Verification items for this drawing (mm, ordinates from the low corner). Give positions to 0.01 mm unless a question says otherwise; leave off trailing zeros. Order: outer loops, then holes, each group sorted by start corner. A loop starts at its lowest first (then second) coordinate and runs counter-clockwise, first axis right, second up. Notation, with made-up numbers: M 74.5,-23 L 83.5,-23 A25 cw 83.5,9 Z; hole C -34.5,3.5 d5. An arc over 180 degrees is marked long. Answer as a JSON object with one key per item and string values.
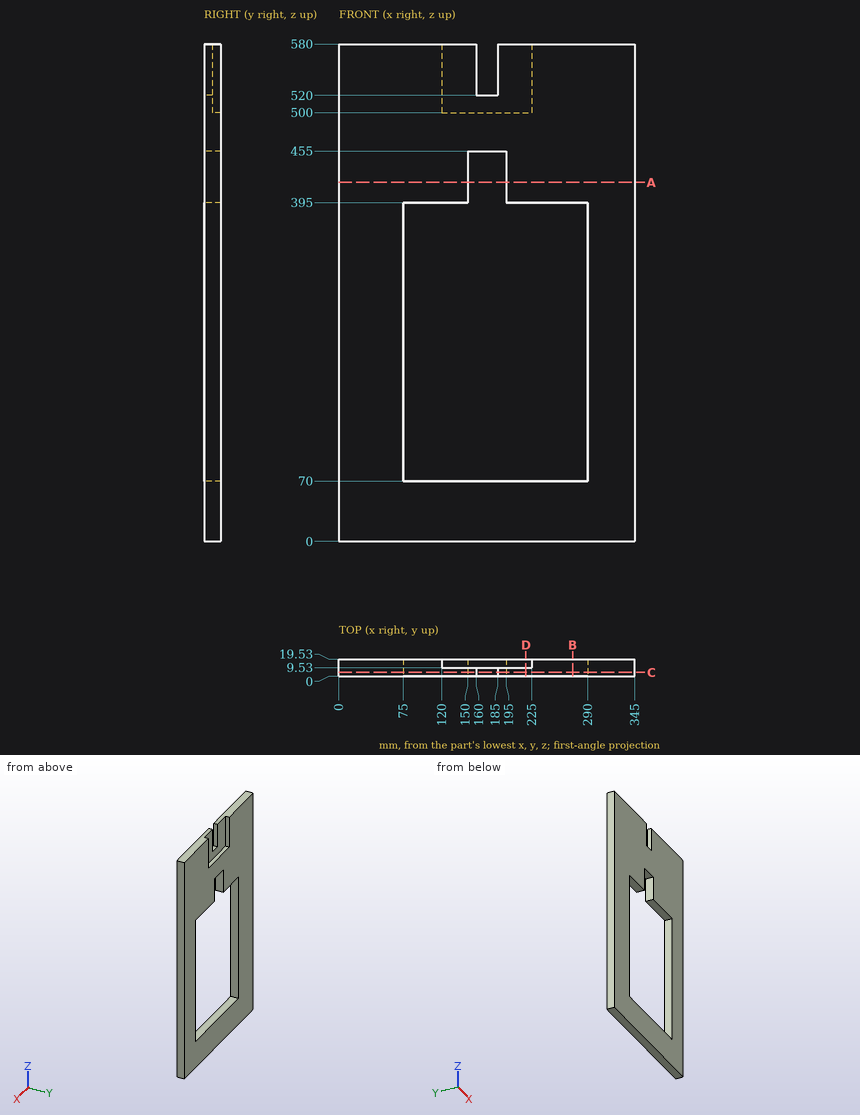
Q1. Material ranges on L1, parallel to Z at x = 204, y = 12.75; L2, parallel to Z at x = 90, y = 1; L3, parallel to X at y = 5, z = 333.5, recorded low to high.
Resolved:
{"L1": "z = 0 to 70, 395 to 500", "L2": "z = 0 to 70, 395 to 580", "L3": "x = 0 to 75, 290 to 345"}
Q2. Gauge pin test, flat ends, axial feed: pin 1 Ø5 at (x, y) = (169.5, 4) entering from +Z; pin 2 Ø6 at (x, y) = (224.5, 15.5) entering from +Z; pin 3 Ø24 at (x, z) = (162.5, 527.5) entering from +Y; pin 4 Ø3 at (x, y) = (163.5, 15) entering from +Z. Record the tip position at first contact, or that the pin passes through.
Resolved:
{"pin 1": "stops at z = 520", "pin 2": "stops at z = 580", "pin 3": "stops at y = 9.53", "pin 4": "stops at z = 500"}
Q3. Section check A-A on z = 418.5. Record the cut outline in (x, y), then the cut area to 3 significant figures.
Resolved:
{"outline": "M 0,0 L 150,0 L 150,19.53 L 0,19.53 Z; M 195,0 L 345,0 L 345,19.53 L 195,19.53 Z", "area": "5,860 mm²"}
Q4. Section check D-D on x = 218. Record the cut outline in (y, z).
Resolved:
{"outline": "M 0,0 L 19.53,0 L 19.53,70 L 0,70 Z; M 0,395 L 19.53,395 L 19.53,500 L 9.53,500 L 9.53,580 L 0,580 Z"}
Q5. Section check C-C on y = 4.25. Record the cut outline in (x, z).
Resolved:
{"outline": "M 0,0 L 345,0 L 345,580 L 185,580 L 185,520 L 160,520 L 160,580 L 0,580 Z; hole M 75,70 L 290,70 L 290,395 L 195,395 L 195,455 L 150,455 L 150,395 L 75,395 Z"}
Q6. Section check B-B on x = 272.5. Record the cut outline in (y, z).
Resolved:
{"outline": "M 0,0 L 19.53,0 L 19.53,70 L 0,70 Z; M 0,395 L 19.53,395 L 19.53,580 L 0,580 Z"}
